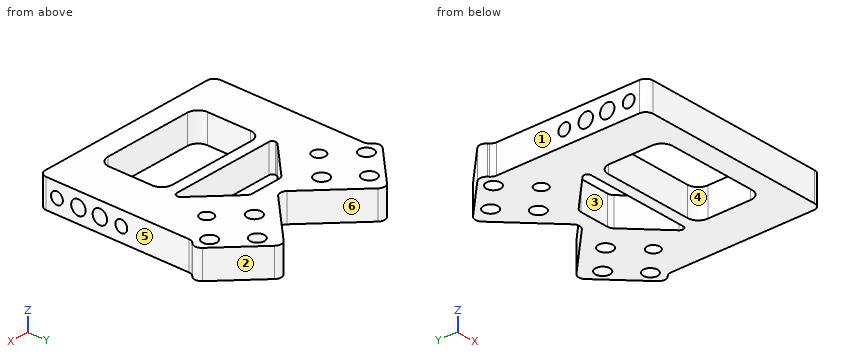
```python
from build123d import *
from OCP.BRepFilletAPI import BRepFilletAPI_MakeFillet

# Parameters (mm, degrees)
SKETCH_1_W          = 55
SKETCH_1_H          = 48
EXTRUDE_1_DEPTH     = 8
SKETCH_2_R          = 1.65
SKETCH_2_R_2        = 2.01
CUT_EXTRUDE_1_DEPTH = 10
SKETCH_4_W          = 5
SKETCH_4_H          = 18
EXTRUDE_2_DEPTH     = 8
CUT_EXTRUDE_2_DEPTH = 8
SKETCH_5_R          = 1.25
CUT_EXTRUDE_3_DEPTH = 8
SKETCH_6_W          = 31
SKETCH_6_H          = 18
CUT_EXTRUDE_4_DEPTH = 8
FILLET_1_R1         = 2
FILLET_1_R2         = 3
FILLET_1_R3         = 5
SKETCH_7_R          = 1.25
EXTRUDE_3_DEPTH     = 8
EXTRUDE_START       = -8
EXTRUDE_4_DEPTH     = 8
CUT_EXTRUDE_START   = -10
CUT_EXTRUDE_6_DEPTH = 10
CUT_EXTRUDE_7_DEPTH = 10
FILLET_4_R          = 2
FILLET_5_R          = 2
FILLET_6_R          = 2
FILLET_7_R          = 1
FILLET_8_R          = 2
SKETCH_13_R         = 2
SKETCH_13_R_2       = 1.793563064
CUT_EXTRUDE_8_DEPTH = 10


with BuildPart() as part:
    # 草图1 → 凸台-拉伸1 (new body)
    with BuildSketch(Plane.XY):
        Rectangle(SKETCH_1_W, SKETCH_1_H)
    extrude(amount=EXTRUDE_1_DEPTH)

    # 草图2 → 切除-拉伸1 (cut)
    with BuildSketch(Plane.ZY.offset(27.5)):
        with Locations((4, -19)):
            Circle(SKETCH_2_R)
        with Locations((4, -1)):
            Circle(SKETCH_2_R)
        with Locations((4, -13)):
            Circle(SKETCH_2_R_2)
        with Locations((4, -7)):
            Circle(SKETCH_2_R_2)
    cut_extrude_1 = extrude(amount=-CUT_EXTRUDE_1_DEPTH, mode=Mode.SUBTRACT)

    # 镜向1: 切除-拉伸1 across plane
    add(cut_extrude_1.mirror(Plane(origin=(0, 0, 0), x_dir=(0, 0, 1), z_dir=(1, 0, 0))), mode=Mode.SUBTRACT)

    # 草图4 → 凸台-拉伸2 (add)
    with BuildSketch(Plane.XY.offset(8)):
        with Locations((30, 15)):
            Rectangle(SKETCH_4_W, SKETCH_4_H)
        with Locations((-30, 15)):
            Rectangle(SKETCH_4_W, SKETCH_4_H)
    extrude(amount=-EXTRUDE_2_DEPTH)

    # 草图3 → 切除-拉伸2 (cut)
    with BuildSketch(Plane.XY.offset(8)):
        Polygon((-32.5, 11.340620434), (-19.840620434, 24), (-32.5, 24), align=None)
        Polygon((32.5, 24), (19.840620434, 24), (32.5, 11.340620434), align=None)
    extrude(amount=-CUT_EXTRUDE_2_DEPTH, mode=Mode.SUBTRACT)

    # 草图5 → 切除-拉伸3 (cut)
    with BuildSketch(Plane.XY.offset(8)):
        with Locations((19.084414101, 19.071067812)):
            Circle(SKETCH_5_R)
        with Locations((26.155481913, 12)):
            Circle(SKETCH_5_R)
        with Locations((19.084414101, 4.928932188)):
            Circle(SKETCH_5_R)
        with Locations((12.013346289, 12)):
            Circle(SKETCH_5_R)
        with Locations(Location((-12.013346289, 12, 0), (0, 0, 180))):
            Circle(SKETCH_5_R)
        with Locations(Location((-19.084414101, 4.928932188, 0), (0, 0, 180))):
            Circle(SKETCH_5_R)
        with Locations(Location((-26.155481913, 12, 0), (0, 0, 180))):
            Circle(SKETCH_5_R)
        with Locations(Location((-19.084414101, 19.071067812, 0), (0, 0, 180))):
            Circle(SKETCH_5_R)
        Polygon((14.841773414, 12), (19.084414101, 16.242640687), (23.327054788, 12), (19.084414101, 7.757359313), align=None)
        Polygon((-19.084414101, 16.242640687), (-23.327054788, 12), (-19.084414101, 7.757359313), (-14.841773414, 12), align=None)
    extrude(amount=-CUT_EXTRUDE_3_DEPTH, mode=Mode.SUBTRACT)

    # 草图6 → 切除-拉伸4 (cut)
    with BuildSketch(Plane.XY.offset(8)):
        with Locations((0, -9)):
            Rectangle(SKETCH_6_W, SKETCH_6_H)
        Polygon((-19.840620434, 24), (0, 4.159379566), (19.840620434, 24), align=None)
        Polygon((32.5, 11.340620434), (27.5, 6), (32.5, 6), align=None)
        Polygon((-32.5, 11.340620434), (-32.5, 6), (-27.5, 6), align=None)
    extrude(amount=-CUT_EXTRUDE_4_DEPTH, mode=Mode.SUBTRACT)

    # 圆角1: one fillet with a radius per group of edges: ONE call of the kernel's fillet builder (fillet() takes one radius for all edges)
    fillet_1_edges_1 = [part.edges().sort_by_distance(p)[0] for p in [
        (-27.5, -24, 4),
        (27.5, -24, 4),
        (-19.084414101, 16.242640687, 4),
        (-14.841773414, 12, 4),
        (-23.327054788, 12, 4),
        (-19.084414101, 7.757359313, 4),
        (14.841773414, 12, 4),
        (19.084414101, 7.757359313, 4),
        (23.327054788, 12, 4),
        (19.084414101, 16.242640687, 4),
    ]]
    fillet_1_edges_2 = [part.edges().sort_by_distance(p)[0] for p in [
        (32.5, 11.340620434, 4),
        (19.840620434, 24, 4),
        (-19.840620434, 24, 4),
        (-32.5, 11.340620434, 4),
        (-27.5, 6, 4),
        (27.5, 6, 4),
        (15.5, 0, 4),
        (-15.5, 0, 4),
        (-15.5, -18, 4),
        (15.5, -18, 4),
    ]]
    fillet_1_edges_3 = [part.edges().sort_by_distance(p)[0] for p in [
        (0, 4.159379566, 4),
    ]]
    fillet_1 = BRepFilletAPI_MakeFillet(part.part.solid().wrapped)
    for e in fillet_1_edges_1:
        fillet_1.Add(FILLET_1_R1, e.wrapped)
    for e in fillet_1_edges_2:
        fillet_1.Add(FILLET_1_R2, e.wrapped)
    for e in fillet_1_edges_3:
        fillet_1.Add(FILLET_1_R3, e.wrapped)
    add(Compound.cast(fillet_1.Shape()), mode=Mode.REPLACE)

    # 草图7 → 凸台-拉伸3 (add)
    with BuildSketch(Plane.XY.offset(8)):
        with Locations((19.084414101, 19.071067812)):
            Circle(SKETCH_7_R)
        with Locations((-26.155481913, 12)):
            Circle(SKETCH_7_R)
        with Locations((-19.084414101, 4.928932188)):
            Circle(SKETCH_7_R)
        with Locations((-19.084414101, 19.071067812)):
            Circle(SKETCH_7_R)
        with Locations((-12.013346289, 12)):
            Circle(SKETCH_7_R)
        with Locations((12.013346289, 12)):
            Circle(SKETCH_7_R)
        with Locations((19.084414101, 4.928932188)):
            Circle(SKETCH_7_R)
        with Locations((26.155481913, 12)):
            Circle(SKETCH_7_R)
        with BuildLine():
            Line((-16.255986976, 13.414213562), (-17.670200539, 14.828427125))
            ThreePointArc((-17.670200539, 14.828427125), (-19.084414101, 15.414213562), (-20.498627663, 14.828427125))
            Line((-20.498627663, 14.828427125), (-21.912841226, 13.414213562))
            ThreePointArc((-21.912841226, 13.414213562), (-22.498627663, 12), (-21.912841226, 10.585786438))
            Line((-21.912841226, 10.585786438), (-20.498627663, 9.171572875))
            ThreePointArc((-20.498627663, 9.171572875), (-19.084414101, 8.585786438), (-17.670200539, 9.171572875))
            Line((-17.670200539, 9.171572875), (-16.255986976, 10.585786438))
            ThreePointArc((-16.255986976, 10.585786438), (-15.670200539, 12), (-16.255986976, 13.414213562))
        make_face()
        with BuildLine():
            Line((16.255986976, 10.585786438), (17.670200539, 9.171572875))
            ThreePointArc((17.670200539, 9.171572875), (19.084414101, 8.585786438), (20.498627663, 9.171572875))
            Line((20.498627663, 9.171572875), (21.912841226, 10.585786438))
            ThreePointArc((21.912841226, 10.585786438), (22.498627663, 12), (21.912841226, 13.414213562))
            Line((21.912841226, 13.414213562), (20.498627663, 14.828427125))
            ThreePointArc((20.498627663, 14.828427125), (19.084414101, 15.414213562), (17.670200539, 14.828427125))
            Line((17.670200539, 14.828427125), (16.255986976, 13.414213562))
            ThreePointArc((16.255986976, 13.414213562), (15.670200539, 12), (16.255986976, 10.585786438))
        make_face()
    extrude(amount=-EXTRUDE_3_DEPTH)

    # 草图9 → 凸台-拉伸4 (add)
    with BuildSketch(Plane.XY.offset(8).offset(EXTRUDE_START)):
        with BuildLine():
            ThreePointArc((30.447405477, 13.393214957), (31.325678544, 11.32128458), (30.516094042, 9.221562694))
            Line((30.516094042, 9.221562694), (36.103109797, 14.808578449))
            Line((36.103109797, 14.808578449), (16.305086528, 34.606601718))
            Line((16.305086528, 34.606601718), (0, 18.30151519))
            Line((0, 18.30151519), (0, 6.230447378))
            ThreePointArc((0, 6.230447378), (1.913417162, 6.611049716), (3.535533906, 7.694913472))
            Line((3.535533906, 7.694913472), (17.71930009, 21.878679656))
            ThreePointArc((17.71930009, 21.878679656), (19.840620434, 22.757359313), (21.961940777, 21.878679656))
            Line((21.961940777, 21.878679656), (30.447405477, 13.393214957))
        make_face()
        with BuildLine():
            Line((0, 6.230447378), (0, 18.30151519))
            Line((0, 18.30151519), (-16.305086528, 34.606601718))
            Line((-16.305086528, 34.606601718), (-36.103109797, 14.808578449))
            Line((-36.103109797, 14.808578449), (-30.516094042, 9.221562694))
            ThreePointArc((-30.516094042, 9.221562694), (-31.325678544, 11.32128458), (-30.447405477, 13.393214957))
            Line((-30.447405477, 13.393214957), (-21.961940777, 21.878679656))
            ThreePointArc((-21.961940777, 21.878679656), (-19.840620434, 22.757359313), (-17.71930009, 21.878679656))
            Line((-17.71930009, 21.878679656), (-3.535533906, 7.694913472))
            ThreePointArc((-3.535533906, 7.694913472), (-1.913417162, 6.611049716), (0, 6.230447378))
        make_face()
    extrude(amount=EXTRUDE_4_DEPTH)

    # 草图10 → 切除-拉伸6 (cut)
    with BuildSketch(Plane.XY.offset(8).offset(CUT_EXTRUDE_START)):
        with BuildLine():
            Line((27.5, 18.756314603), (27.5, 4.814839075))
            ThreePointArc((27.5, 4.814839075), (27.70983632, 5.917103398), (28.309991091, 6.865170995))
            Line((28.309991091, 6.865170995), (30.516094042, 9.221562694))
            Line((30.516094042, 9.221562694), (36.103109797, 14.808578449))
            Line((36.103109797, 14.808578449), (29.827686821, 21.084001424))
            Line((29.827686821, 21.084001424), (27.5, 18.756314603))
        make_face()
        with BuildLine():
            ThreePointArc((-28.309991091, 6.865170995), (-27.70983632, 5.917103398), (-27.5, 4.814839075))
            Line((-27.5, 4.814839075), (-27.5, 18.756314603))
            Line((-27.5, 18.756314603), (-29.827686821, 21.084001424))
            Line((-29.827686821, 21.084001424), (-36.103109797, 14.808578449))
            Line((-36.103109797, 14.808578449), (-30.516094042, 9.221562694))
            Line((-30.516094042, 9.221562694), (-28.309991091, 6.865170995))
        make_face()
    extrude(amount=CUT_EXTRUDE_6_DEPTH, mode=Mode.SUBTRACT)

    # 草图11 → 切除-拉伸7 (cut)
    with BuildSketch(Plane.XY.offset(8)):
        Polygon((-5, 15), (-15.5, 4.5), (-15.5, 3), (15.5, 3), (15.5, 4.5), (5, 15), align=None)
    extrude(amount=-CUT_EXTRUDE_7_DEPTH, mode=Mode.SUBTRACT)

    # 圆角4
    fillet_4_edges = [part.edges().sort_by_distance(p)[0] for p in [
        (-27.5, 18.756314603, 4),
    ]]
    fillet(fillet_4_edges, radius=FILLET_4_R)

    # 圆角5
    fillet_5_edges = [part.edges().sort_by_distance(p)[0] for p in [
        (-16.305086528, 34.606601718, 4),
        (16.305086528, 34.606601718, 4),
        (0, 18.30151519, 4),
        (29.827686821, 21.084001424, 4),
        (-29.827686821, 21.084001424, 4),
    ]]
    fillet(fillet_5_edges, radius=FILLET_5_R)

    # 圆角6
    fillet_6_edges = [part.edges().sort_by_distance(p)[0] for p in [
        (27.5, 18.756314603, 4),
    ]]
    fillet(fillet_6_edges, radius=FILLET_6_R)

    # 圆角7
    fillet_7_edges = [part.edges().sort_by_distance(p)[0] for p in [
        (15.5, 4.5, 4),
        (15.5, 3, 4),
        (-15.5, 3, 4),
        (-15.5, 4.5, 4),
    ]]
    fillet(fillet_7_edges, radius=FILLET_7_R)

    # 圆角8
    fillet_8_edges = [part.edges().sort_by_distance(p)[0] for p in [
        (-5, 15, 4),
        (5, 15, 4),
    ]]
    fillet(fillet_8_edges, radius=FILLET_8_R)

    # 草图13 → 切除-拉伸8 (cut)
    with BuildSketch(Plane.XY.offset(8)):
        with Locations((17.67766953, 28.302433917)):
            Circle(SKETCH_13_R)
        with Locations((24.748737342, 21.231366105)):
            Circle(SKETCH_13_R)
        with Locations((17.67766953, 14.160298293)):
            Circle(SKETCH_13_R_2)
        with Locations((10.606601718, 21.231366105)):
            Circle(SKETCH_13_R)
        with Locations((-10.606601718, 21.231366105)):
            Circle(SKETCH_13_R)
        with Locations((-17.67766953, 14.160298293)):
            Circle(SKETCH_13_R_2)
        with Locations((-24.748737342, 21.231366105)):
            Circle(SKETCH_13_R)
        with Locations((-17.67766953, 28.302433917)):
            Circle(SKETCH_13_R)
    extrude(amount=-CUT_EXTRUDE_8_DEPTH, mode=Mode.SUBTRACT)


solid = part.part
```
CAD build for the part. Positions are in the model's coordinates, mm. Face numbers are marked on the shaded views. A direction names the side the tool comes from. Round coordinates to 2 decimals unless told otherwise and drop trailing zeros. Order: outer loops, then holes, each group sorted by start corner. A loop starts at its lowest first (then second) coordinate and runs counter-clockwise, first axis right, second up. Notation, with made-up numbers: (74.5, 66.25) -> (97.5, 66.25) arc R29 ccw to (97.5, 100.25) -> close; hole circle Ø7 at (53, -33). An arc over 180 degrees is marked (long way). Write item = value, one per line.
(1) 3-axis set-ups, long thin cutter, end or side, ignore diameter. For the marked faces 4, 5 and 6: which of +Z, -Z, +X, -X, +Y, -Y reach the whole face in a straight line?
Answers follow:
face_4 = +Z, -Z
face_5 = +Z, -Z, +X, -Y
face_6 = +Z, -Z, +Y
(2) Cut at C-C (z = 4.25). State how many separate pieces and enclosed holes the cut face has, plus the area to 3 significant figures.
Answers follow:
separate_pieces = 1
enclosed_holes = 10
area = 1,640 mm²
(3) Flat gauge pins, fed straight in: P1, Ø4.5, axis at y = -13.5, z = 4.5, coming from the +X side; P2, Ø1.6, axis at y = -18.5, z = 4, coming from the -X side; P3, Ø2.5, axis at y = -12, z = 3.5, coming from the -X side; P4, Ø5, axis at x = -2, y = 11.5, coming from the +Z side. Where does each tip first touch, or does it go through?
Answers follow:
P1 = 27.5
P2 = -17.5
P3 = -27.5
P4 = through
(4) Cut at B-B (y = -1). Write the cut outline in (x, z).
Answers follow:
outline = (-27.5, 0) -> (-14.74, 0) -> (-14.74, 8) -> (-27.5, 8) -> (-27.5, 5.65) -> (-17.5, 5.65) -> (-17.5, 2.35) -> (-27.5, 2.35) -> close; (14.74, 0) -> (27.5, 0) -> (27.5, 2.35) -> (17.5, 2.35) -> (17.5, 5.65) -> (27.5, 5.65) -> (27.5, 8) -> (14.74, 8) -> close
(5) Pull direction X, two halves, no side cores. Call the marked faces 1, 2 and 3: +X half, -X half, draft (parallel to the pull), parting line (faces both ways), or undercut.
Answers follow:
face_1 = -X half
face_2 = +X half
face_3 = undercut
(6) Cut at A-A (y = -13). Write the cut outline in (x, z).
Answers follow:
outline = (-27.5, 0) -> (-15.5, 0) -> (-15.5, 8) -> (-27.5, 8) -> (-27.5, 6.01) -> (-17.5, 6.01) -> (-17.5, 1.99) -> (-27.5, 1.99) -> close; (15.5, 0) -> (27.5, 0) -> (27.5, 1.99) -> (17.5, 1.99) -> (17.5, 6.01) -> (27.5, 6.01) -> (27.5, 8) -> (15.5, 8) -> close
(7) Drill centre lines: L1, parallel to X at y = 14, z = 2; L2, parallel to Y at x = -9, z = 5.75; L3, parallel to Y at x = -13, z = 2.5. Where is each one in solid material? Low to high.
Answers follow:
L1 = -27.5 to -19.46, -15.89 to -6, 6 to 15.89, 19.46 to 27.5
L2 = -24 to -18, 0 to 3, 11 to 20.04, 22.42 to 27.3
L3 = -24 to -17.96, -0.04 to 3, 7 to 31.3
